```python
from build123d import *

# Parameters (mm, degrees)
SKETCH_1_R      = 3
SKETCH_1_R_2    = 5.05
SKETCH_1_R_3    = 2.05
EXTRUDE_2_DEPTH = 2
FILLET_1_R      = 1.3


with BuildPart() as part:
    # 草图1 → 凸台-拉伸2 (new body)
    with BuildSketch(Plane.XY):
        with BuildLine():
            Line((-55.962487977, 23.496493589), (-55.962487977, 8.046493589))
            Line((-55.962487977, 8.046493589), (-51.962487977, 8.046493589))
            Line((-51.962487977, 8.046493589), (-51.962487977, 9.496493589))
            Line((-51.962487977, 9.496493589), (-48.762487977, 9.496493589))
            Line((-48.762487977, 9.496493589), (-48.762487977, 8.046493589))
            Line((-48.762487977, 8.046493589), (-45.562487977, 8.046493589))
            Line((-45.562487977, 8.046493589), (-45.562487977, 3.946493589))
            Line((-45.562487977, 3.946493589), (-48.762487977, 3.946493589))
            Line((-48.762487977, 3.946493589), (-48.762487977, 2.496493589))
            Line((-48.762487977, 2.496493589), (-51.962487977, 2.496493589))
            Line((-51.962487977, 2.496493589), (-51.962487977, 3.946493589))
            Line((-51.962487977, 3.946493589), (-55.962487977, 3.946493589))
            Line((-55.962487977, 3.946493589), (-55.962487977, -5.003506411))
            Line((-55.962487977, -5.003506411), (-60.962487977, -5.003506411))
            Line((-60.962487977, -5.003506411), (-60.962487977, -13.003506411))
            Line((-60.962487977, -13.003506411), (-55.962487977, -13.003506411))
            Line((-55.962487977, -13.003506411), (-55.962487977, -21.953506411))
            Line((-55.962487977, -21.953506411), (-51.962487977, -21.953506411))
            Line((-51.962487977, -21.953506411), (-51.962487977, -20.503506411))
            Line((-51.962487977, -20.503506411), (-48.762487977, -20.503506411))
            Line((-48.762487977, -20.503506411), (-48.762487977, -21.953506411))
            Line((-48.762487977, -21.953506411), (-45.562487977, -21.953506411))
            Line((-45.562487977, -21.953506411), (-45.562487977, -26.053506411))
            Line((-45.562487977, -26.053506411), (-48.762487977, -26.053506411))
            Line((-48.762487977, -26.053506411), (-48.762487977, -27.503506411))
            Line((-48.762487977, -27.503506411), (-51.962487977, -27.503506411))
            Line((-51.962487977, -27.503506411), (-51.962487977, -26.053506411))
            Line((-51.962487977, -26.053506411), (-55.962487977, -26.053506411))
            Line((-55.962487977, -26.053506411), (-55.962487977, -35.003506411))
            Line((-55.962487977, -35.003506411), (-60.962487977, -35.003506411))
            Line((-60.962487977, -35.003506411), (-60.962487977, -43.003506411))
            Line((-60.962487977, -43.003506411), (-55.962487977, -43.003506411))
            Line((-55.962487977, -43.003506411), (-55.962487977, -51.953506411))
            Line((-55.962487977, -51.953506411), (-51.962487977, -51.953506411))
            Line((-51.962487977, -51.953506411), (-51.962487977, -50.503506411))
            Line((-51.962487977, -50.503506411), (-48.762487977, -50.503506411))
            Line((-48.762487977, -50.503506411), (-48.762487977, -51.953506411))
            Line((-48.762487977, -51.953506411), (-45.562487977, -51.953506411))
            Line((-45.562487977, -51.953506411), (-45.562487977, -56.053506411))
            Line((-45.562487977, -56.053506411), (-48.762487977, -56.053506411))
            Line((-48.762487977, -56.053506411), (-48.762487977, -57.503506411))
            Line((-48.762487977, -57.503506411), (-51.962487977, -57.503506411))
            Line((-51.962487977, -57.503506411), (-51.962487977, -56.053506411))
            Line((-51.962487977, -56.053506411), (-55.962487977, -56.053506411))
            Line((-55.962487977, -56.053506411), (-55.962487977, -61.503506411))
            Line((-55.962487977, -61.503506411), (-67.962487977, -61.503506411))
            Line((-67.962487977, -61.503506411), (-67.962487977, -65.791888255))
            Line((-67.962487977, -65.791888255), (38.037512023, -65.791888255))
            Line((38.037512023, -65.791888255), (38.037512023, -61.503506411))
            Line((38.037512023, -61.503506411), (26.037512023, -61.503506411))
            Line((26.037512023, -61.503506411), (26.037512023, -56.053506411))
            Line((26.037512023, -56.053506411), (22.037512023, -56.053506411))
            Line((22.037512023, -56.053506411), (22.037512023, -57.503506411))
            Line((22.037512023, -57.503506411), (18.837512023, -57.503506411))
            Line((18.837512023, -57.503506411), (18.837512023, -56.053506411))
            Line((18.837512023, -56.053506411), (15.637512023, -56.053506411))
            Line((15.637512023, -56.053506411), (15.637512023, -51.953506411))
            Line((15.637512023, -51.953506411), (18.837512023, -51.953506411))
            Line((18.837512023, -51.953506411), (18.837512023, -50.503506411))
            Line((18.837512023, -50.503506411), (22.037512023, -50.503506411))
            Line((22.037512023, -50.503506411), (22.037512023, -51.953506411))
            Line((22.037512023, -51.953506411), (26.037512023, -51.953506411))
            Line((26.037512023, -51.953506411), (26.037512023, -43.003506411))
            Line((26.037512023, -43.003506411), (31.037512023, -43.003506411))
            Line((31.037512023, -43.003506411), (31.037512023, -35.003506411))
            Line((31.037512023, -35.003506411), (26.037512023, -35.003506411))
            Line((26.037512023, -35.003506411), (26.037512023, -26.053506411))
            Line((26.037512023, -26.053506411), (22.037512023, -26.053506411))
            Line((22.037512023, -26.053506411), (22.037512023, -27.503506411))
            Line((22.037512023, -27.503506411), (18.837512023, -27.503506411))
            Line((18.837512023, -27.503506411), (18.837512023, -26.053506411))
            Line((18.837512023, -26.053506411), (15.637512023, -26.053506411))
            Line((15.637512023, -26.053506411), (15.637512023, -21.953506411))
            Line((15.637512023, -21.953506411), (18.837512023, -21.953506411))
            Line((18.837512023, -21.953506411), (18.837512023, -20.503506411))
            Line((18.837512023, -20.503506411), (22.037512023, -20.503506411))
            Line((22.037512023, -20.503506411), (22.037512023, -21.953506411))
            Line((22.037512023, -21.953506411), (26.037512023, -21.953506411))
            Line((26.037512023, -21.953506411), (26.037512023, -13.003506411))
            Line((26.037512023, -13.003506411), (31.037512023, -13.003506411))
            Line((31.037512023, -13.003506411), (31.037512023, -5.003506411))
            Line((31.037512023, -5.003506411), (26.037512023, -5.003506411))
            Line((26.037512023, -5.003506411), (26.037512023, 3.946493589))
            Line((26.037512023, 3.946493589), (22.037512023, 3.946493589))
            Line((22.037512023, 3.946493589), (22.037512023, 2.496493589))
            Line((22.037512023, 2.496493589), (18.837512023, 2.496493589))
            Line((18.837512023, 2.496493589), (18.837512023, 3.946493589))
            Line((18.837512023, 3.946493589), (15.637512023, 3.946493589))
            Line((15.637512023, 3.946493589), (15.637512023, 8.046493589))
            Line((15.637512023, 8.046493589), (18.837512023, 8.046493589))
            Line((18.837512023, 8.046493589), (18.837512023, 9.496493589))
            Line((18.837512023, 9.496493589), (22.037512023, 9.496493589))
            Line((22.037512023, 9.496493589), (22.037512023, 8.046493589))
            Line((22.037512023, 8.046493589), (26.037512023, 8.046493589))
            Line((26.037512023, 8.046493589), (26.037512023, 23.496493589))
            Line((26.037512023, 23.496493589), (26.037512023, 31.722989041))
            ThreePointArc((26.037512023, 31.722989041), (-14.962487977, 51.269592797), (-55.962487977, 31.722989041))
            Line((-55.962487977, 31.722989041), (-55.962487977, 23.496493589))
        make_face()
        with Locations((-14.962487977, -25.253506411)):
            Circle(SKETCH_1_R, mode=Mode.SUBTRACT)
        with Locations((4.523083608, -12.753506411)):
            Circle(SKETCH_1_R, mode=Mode.SUBTRACT)
        with Locations((-14.962487977, -1.503506411)):
            Circle(SKETCH_1_R_2, mode=Mode.SUBTRACT)
        with Locations((-35.530591317, 10.371493589)):
            Circle(SKETCH_1_R, mode=Mode.SUBTRACT)
        with Locations((-34.448059562, -12.753506411)):
            Circle(SKETCH_1_R, mode=Mode.SUBTRACT)
        with Locations((5.605615363, 10.371493589)):
            Circle(SKETCH_1_R, mode=Mode.SUBTRACT)
        with Locations((-14.962487977, 20.996493589)):
            Circle(SKETCH_1_R, mode=Mode.SUBTRACT)
        with Locations((18.271530739, -34.737525127)):
            Circle(SKETCH_1_R_3, mode=Mode.SUBTRACT)
        with Locations((-14.962487977, -48.503506411)):
            Circle(SKETCH_1_R_3, mode=Mode.SUBTRACT)
        with Locations((-48.196506692, -34.737525127)):
            Circle(SKETCH_1_R_3, mode=Mode.SUBTRACT)
        with Locations((-48.196506692, 31.730512305)):
            Circle(SKETCH_1_R_3, mode=Mode.SUBTRACT)
        with Locations((-14.962487977, 45.496493589)):
            Circle(SKETCH_1_R_3, mode=Mode.SUBTRACT)
        with Locations((18.271530739, 31.730512305)):
            Circle(SKETCH_1_R_3, mode=Mode.SUBTRACT)
    extrude(amount=EXTRUDE_2_DEPTH)

    # 圆角1
    fillet_1_edges = [part.edges().sort_by_distance(p)[0] for p in [
        (-60.962487977, -43.003506411, 1),
        (-60.962487977, -35.003506411, 1),
        (-60.962487977, -13.003506411, 1),
        (-60.962487977, -5.003506411, 1),
        (31.037512023, -5.003506411, 1),
        (31.037512023, -13.003506411, 1),
        (31.037512023, -35.003506411, 1),
        (31.037512023, -43.003506411, 1),
    ]]
    fillet(fillet_1_edges, radius=FILLET_1_R)


solid = part.part
```
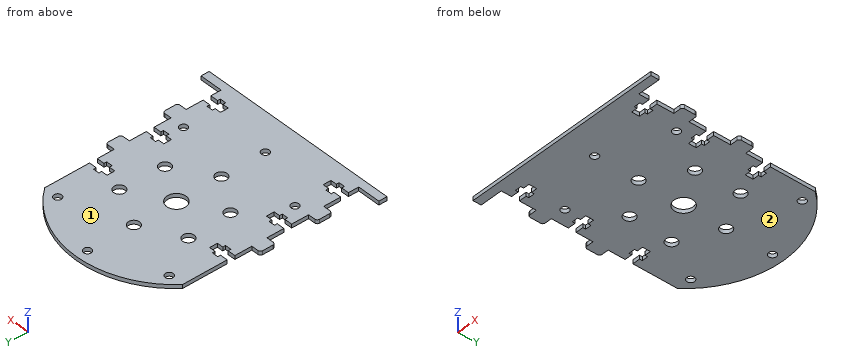
Model file for the job. Use its own axes, mm. Face numbers are marked on the shaded views. Coordinates: 2 decimals unless noted, no trailing zeros. Loops run counter-clockwise (first coordinate to the right, second up) from the corner with the lowest first, then second, coordinate; pieces in that order, holes last. Notation, with made-up numbers: M 53.25,31.5 L 67.25,31.5 A23 ccw 67.25,56.5 Z; hole C 9.25,12 d8. An arc over 180 degrees is marked long. Use CSV: the item, a comma, the result in double quotes. Start each with the question number.
1. Probe probe 1 along X at (y, z) = (-34.5, 0.55); probe 2 along X at (y, z) = (-21, 1.25); probe 3 along Y at (x, z) = (-57, 0.85). List the from-to ranges inside material, lowest first. Write a range as [from, to].
2. Band-saw the part on A-A, the plane y = -17.5. List the corners of the cut face in (x, z), then the cut area to 3 significant figures.
3. Band-saw the part on C-C, the plane z = 1.4. Give the number of separate pieces and of enclosed holes in the cut face, then the cut area to 3 significant figures.
4. Flat gauge pins, fed straight in: pin 1 (0.6 mm diameter, centred on y = -2.5, z = 1.5, fed in from -X); pin 2 (3.5 mm diameter, centred on x = -48.2, y = -34.74, fed in from +Z); pin 3 (7 mm diameter, centred on x = 4.52, y = -12.75, fed in from +Z); pin 4 (1 mm diameter, centred on y = 18, z = 1.5, fed in from +X). Where does each tip first touch, or does it go through?
5. Band-saw the part on B-B, the plane x = 12.5. List the corners of the cut face in (y, z), then the cut area to 3 significant figures.
6. Two-plate mould, pull along Z, no slides. Class the marked faces 1 and 2: pulls with the +Z half, pulls with the -Z half, needs draft (parallel to the pull), parting line crosses it, or undercut.
Entries:
1,probe 1,"x = [-55.96, -50.23], [-46.16, 16.24], [20.31, 26.04]"
1,probe 2,"x = [-55.96, -51.96], [-48.76, 18.84], [22.04, 26.04]"
1,probe 3,"y = [-65.79, -61.5], [-43, -35], [-13, -5]"
2,outline,"M -55.96,0 L 26.04,0 L 26.04,2 L -55.96,2 Z"
2,area,"164 mm2"
3,separate pieces,"1"
3,enclosed holes,"13"
3,area,"8,730 mm2"
4,pin 1,"stops at x = -55.96"
4,pin 2,"passes through"
4,pin 3,"stops at z = 2"
4,pin 4,"stops at x = 26.04"
5,outline,"M -65.79,0 L 43.56,0 L 43.56,2 L -65.79,2 Z"
5,area,"219 mm2"
6,face 1,"pulls with the +Z half"
6,face 2,"pulls with the -Z half"
